Here's how the part is built. I have some questions about the finished solid (model axes, mm). A direction names the side the tool comes from. Coordinates: 2 decimals unless noted, no trailing zeros. Loops run counter-clockwise (first coordinate to the right, second up) from the corner with the lowest first, then second, coordinate; pieces in that order, holes last. Notation, with made-up numbers: M 58.25,-5 L 116.25,-5 A20 cw 116.25,19 Z; hole C 32.25,-21.75 d5. An arc over 180 degrees is marked long. Use CSV: the item, a comma, the result in double quotes. Start each with the question number.
Q1. For pin 1 Ø5 at (x, z) = (-4.05, 18.44) entering from +Y; pin 2 Ø4 at (x, y) = (3, -9.5) entering from -Z; pin 3 Ø12 at (y, z) = (0.5, 5.5) entering from +X; pin 4 Ø14 at (x, z) = (0, 0) entering from -Y, each with a flat end and sliding along its axis, tell me the tip position at first contact or that it passes through.
Q2. Please list where these lines run through material, in increasing order: probe 1 along Z at (x, y) = (0, -0.5); probe 2 along Z at (x, y) = (-4, -16.75); probe 3 along Y at (x, z) = (-13, 19). Write a range as [from, to].
Q3. If we section it at B-B (x = 1.25): Please give me the cut outline in (y, z), and give its area (3 significant figures).
Q4. If we section it at A-A (z = -5): Please give me the cut outline in (x, y) (3 decimals).
Q5. If we section it at D-D (y = -16.75): Please give me the cut outline in (x, z).
Q6. If we section it at C-C (y = -9.5): Please give me the cut outline in (x, z), and give its area (3 significant figures).
Q7. If we mould it in two halves opening along Z, with no side actions, what happens to faces 1 (the flat face through (1.71, -17.46, 16.34)), 2 (the flat face through (-10, -17, -8)), 3 (the flat face through (-9, -20, 9))? For each: +Z half, -Z half, draft (parallel to the pull), parting line (faces both ways), or undercut.
Q8. Which directions (+Z, -Z, +X, -X, +Y, -Y) give clear straight access to the entire face, cutting with the end or side of a thin tool? Please do faces 4 (the cylindrical face through (-7.81, -6.75, -1.73)), 5 (the cylindrical face through (-3.12, -17.46, 16.67)).
from build123d import *

# Parameters (mm, degrees)
BOSS_EXTRUDE1_DEPTH      = 30
BOSS_EXTRUDE1_DEPTH_BACK = 20
SKETCH1_R                = 8
SKETCH1_4_R              = 6
SKETCH2_R                = 6
SKETCH1_5_R              = 6
CUT_EXTRUDE1_DEPTH       = 5
BOSS_EXTRUDE3_START      = -5
BOSS_EXTRUDE3_OUTLINE_R  = 2
BOSS_EXTRUDE3_DEPTH      = 5


# Read off the part's stored shape, not the designer's step: Boss-Extrude3
with BuildPart() as part:
    # Sketch1 → Boss-Extrude1 (new, two sides: drawn at the far end of the back side and taken through both)
    with BuildSketch(Plane(origin=(0, 0, 0), x_dir=(1, 0, 0), z_dir=(0, 1, 0)).offset(-BOSS_EXTRUDE1_DEPTH_BACK)):
        with Locations(Location((0, 0, 0), (0, 0, 270))):
            Circle(SKETCH1_R)
    extrude(amount=BOSS_EXTRUDE1_DEPTH + BOSS_EXTRUDE1_DEPTH_BACK)

    # SurfaceCut1
    split(bisect_by=Plane(origin=(0, 0, 0), x_dir=(0, 0, -1), z_dir=(0.6427876096865405, 0.766044443118977, -2.2049215546234306e-15)), keep=Keep.BOTTOM)

    # Sketch1<4> → Cut-Loft1 section 0
    with BuildSketch(Plane(origin=(0, 0, 0), x_dir=(1, 0, 0), z_dir=(0, 1, 0))):
        Circle(SKETCH1_4_R)
    # Sketch2 → Cut-Loft1 section 1
    with BuildSketch(Plane.XZ.offset(20)):
        Circle(SKETCH2_R)
    loft(mode=Mode.SUBTRACT)

    # Sketch1<5> → Cut-Extrude1 (cut)
    with BuildSketch(Plane(origin=(0, 0, 0), x_dir=(1, 0, 0), z_dir=(0, 1, 0))):
        with Locations(Location((0, 0, 0), (0, 0, 90))):
            Circle(SKETCH1_5_R)
    extrude(amount=CUT_EXTRUDE1_DEPTH, mode=Mode.SUBTRACT)

    # Boss-Extrude3 outline → Boss-Extrude3 (add)
    with BuildSketch(Plane.XZ.offset(20).offset(BOSS_EXTRUDE3_START)):
        with BuildLine():
            Line((-20, -8), (0, -8))
            ThreePointArc((0, -8), (-8, 0), (0, 8))
            Line((0, 8), (3.468102534, 24.907883087))
            ThreePointArc((3.468102534, 24.907883087), (-12.594718707, 22.462264233), (-20, 8))
            Line((-20, 8), (-20, -8))
        make_face()
        with Locations((-13.851036571, -1.379219301)):
            Circle(BOSS_EXTRUDE3_OUTLINE_R, mode=Mode.SUBTRACT)
        with Locations((-4.045326452, 18.443425538)):
            Circle(BOSS_EXTRUDE3_OUTLINE_R, mode=Mode.SUBTRACT)
    extrude(amount=BOSS_EXTRUDE3_DEPTH)


solid = part.part
Results below:
1,pin 1,"y = -15"
1,pin 2,"z = -7.94"
1,pin 3,"x = 6.49"
1,pin 4,"y = -20"
2,probe 1,"[-8, -6], [6, 8]"
2,probe 2,"[-8, -4.47], [4.47, 16.44], [20.44, 25.73]"
2,probe 3,"[-20, -15]"
3,outline,"M -20,-7.9 L -1.05,-7.9 L -1.05,-5.87 L -20,-5.87 Z; M -20,5.87 L -1.05,5.87 L -1.05,7.9 L -20,7.9 Z; M -20,14.09 L -15,14.09 L -15,25.49 L -20,25.49 Z"
3,area,"134 mm^2"
4,outline,"M -20,-20 L -3.317,-20 L -3.317,2.783 L -6.245,5.24 L -6.245,-15 L -20,-15 Z; M 3.317,-20 L 6.245,-20 L 6.245,-5.24 L 3.317,-2.783 Z"
5,outline,"M -20,-8 L 0,-8 A8 ccw 0,8 L 3.47,24.91 A17.82 ccw -20,8 Z; hole C -13.85,-1.38 d4; hole C -4.05,18.44 d4; hole C 0,0 d12"
6,outline,"C 0,0 d16; hole C 0,0 d12"
6,area,"88.0 mm^2"
7,face 1,"undercut"
7,face 2,"-Z half"
7,face 3,"draft"
8,face 4,"+Y"
8,face 5,"+Y, -Y"
